from build123d import *

# Parameters (mm, degrees)
SKETCH1_R                     = 3.6195
SKETCH1_R_2                   = 4.7625
SKETCH1_R_3                   = 1.6999966
SKETCH1_W                     = 6.5278
SKETCH1_H                     = 6.5278
BOSS_EXTRUDE1_DEPTH           = 6.35
TAP_DRILL_FOR_6_32_TAP4_D     = 2.7051
TAP_DRILL_FOR_6_32_TAP4_DEPTH = 10.16
TAP_DRILL_FOR_6_32_TAP4_TIP   = 0.81269403
TAP_DRILL_FOR_6_32_TAP3_D     = 2.7051
TAP_DRILL_FOR_6_32_TAP3_DEPTH = 10.16
TAP_DRILL_FOR_6_32_TAP3_TIP   = 0.81269403
SKETCH11_W                    = 6.35
SKETCH11_H                    = 6.1722
BOSS_EXTRUDE2_DEPTH           = 1.016
SKETCH12_W                    = 6.35
SKETCH12_H                    = 6.1722
BOSS_EXTRUDE3_DEPTH           = 1.016
TAP_DRILL_FOR_6_32_TAP1_D     = 2.7051
TAP_DRILL_FOR_6_32_TAP1_DEPTH = 7.62
TAP_DRILL_FOR_6_32_TAP1_TIP   = 0.81269403
TAP_DRILL_FOR_6_32_TAP2_D     = 2.7051
TAP_DRILL_FOR_6_32_TAP2_DEPTH = 7.62
TAP_DRILL_FOR_6_32_TAP2_TIP   = 0.81269403
F_6_CLEARANCE_HOLE1_D         = 3.7973
F_6_CLEARANCE_HOLE1_DEPTH     = 12.7
F_6_CLEARANCE_HOLE1_TIP       = 1.140824014
SKETCH19_R                    = 1.5875
CUT_EXTRUDE1_DEPTH            = 161.894515133
CUT_EXTRUDE2_DEPTH            = 161.894515133


with BuildPart() as part:
    # Sketch1 → Boss-Extrude1 (new body)
    with BuildSketch(Plane(origin=(0, 0, 0), x_dir=(0, 0, -1), z_dir=(1, 0, 0))):
        Polygon((0, 0), (-14.664696837, 25.4), (-144.085303163, 25.4), (-158.75, 0), align=None)
        with Locations((-130.048, 12.7)):
            Circle(SKETCH1_R, mode=Mode.SUBTRACT)
        with Locations((-28.702, 12.7)):
            Circle(SKETCH1_R_2, mode=Mode.SUBTRACT)
        with Locations((-121.5479916, 12.7)):
            Circle(SKETCH1_R_3, mode=Mode.SUBTRACT)
        with Locations((-138.5480084, 12.7)):
            Circle(SKETCH1_R_3, mode=Mode.SUBTRACT)
        with Locations((-79.2861, 12.7889)):
            Rectangle(SKETCH1_W, SKETCH1_H, mode=Mode.SUBTRACT)
    extrude(amount=BOSS_EXTRUDE1_DEPTH)

    # Tap Drill for #6-32 Tap4
    with Locations(Plane(origin=(0, 25.4, 0), x_dir=(1, 0, 0), z_dir=(0, 1, 0))):
        with Locations((3.175, -123.257303163), (3.175, -35.492696837)):
            Hole(TAP_DRILL_FOR_6_32_TAP4_D / 2, depth=TAP_DRILL_FOR_6_32_TAP4_DEPTH)
            with Locations((0, 0, -(TAP_DRILL_FOR_6_32_TAP4_DEPTH + TAP_DRILL_FOR_6_32_TAP4_TIP / 2))):  # 118° drill point
                Cone(0, TAP_DRILL_FOR_6_32_TAP4_D / 2, TAP_DRILL_FOR_6_32_TAP4_TIP, mode=Mode.SUBTRACT)

    # Tap Drill for #6-32 Tap3
    with Locations(Plane(origin=(0, 0, 0), x_dir=(-1, 0, 0), z_dir=(0, -1, 0))):
        with Locations((-3.175, -116.84), (-3.175, -35.56)):
            Hole(TAP_DRILL_FOR_6_32_TAP3_D / 2, depth=TAP_DRILL_FOR_6_32_TAP3_DEPTH)
            with Locations((0, 0, -(TAP_DRILL_FOR_6_32_TAP3_DEPTH + TAP_DRILL_FOR_6_32_TAP3_TIP / 2))):  # 118° drill point
                Cone(0, TAP_DRILL_FOR_6_32_TAP3_D / 2, TAP_DRILL_FOR_6_32_TAP3_TIP, mode=Mode.SUBTRACT)

    # Sketch11 → Boss-Extrude2 (add)
    with BuildSketch(Plane(origin=(0, 68.740766425, 119.0625), x_dir=(1, 0, 0), z_dir=(0, 0.5000000000000038, 0.8660254037844366))):
        with Locations((3.175, -69.9389)):
            Rectangle(SKETCH11_W, SKETCH11_H)
    extrude(amount=BOSS_EXTRUDE2_DEPTH)

    # Sketch12 → Boss-Extrude3 (add)
    with BuildSketch(Plane(origin=(0, 0, 0), x_dir=(-1, 0, 0), z_dir=(0, 0.499999999999998, -0.8660254037844397))):
        with Locations((-3.175, 9.4361)):
            Rectangle(SKETCH12_W, SKETCH12_H)
    extrude(amount=BOSS_EXTRUDE3_DEPTH)

    # Tap Drill for #6-32 Tap1
    with Locations(Plane(origin=(0, 68.740766425, 119.0625), x_dir=(1, 0, 0), z_dir=(0, 0.5000000000000038, 0.8660254037844366))):
        with Locations((3.175, -60.205606325)):
            Hole(TAP_DRILL_FOR_6_32_TAP1_D / 2, depth=TAP_DRILL_FOR_6_32_TAP1_DEPTH)
            with Locations((0, 0, -(TAP_DRILL_FOR_6_32_TAP1_DEPTH + TAP_DRILL_FOR_6_32_TAP1_TIP / 2))):  # 118° drill point
                Cone(0, TAP_DRILL_FOR_6_32_TAP1_D / 2, TAP_DRILL_FOR_6_32_TAP1_TIP, mode=Mode.SUBTRACT)

    # Tap Drill for #6-32 Tap2
    with Locations(Plane(origin=(0, 0, 0), x_dir=(-1, 0, 0), z_dir=(0, 0.49999999999999806, -0.8660254037844398))):
        with Locations((-3.175, 19.169393675)):
            Hole(TAP_DRILL_FOR_6_32_TAP2_D / 2, depth=TAP_DRILL_FOR_6_32_TAP2_DEPTH)
            with Locations((0, 0, -(TAP_DRILL_FOR_6_32_TAP2_DEPTH + TAP_DRILL_FOR_6_32_TAP2_TIP / 2))):  # 118° drill point
                Cone(0, TAP_DRILL_FOR_6_32_TAP2_D / 2, TAP_DRILL_FOR_6_32_TAP2_TIP, mode=Mode.SUBTRACT)

    # #6 Clearance Hole1
    with Locations(Plane(origin=(0, 25.4, 0), x_dir=(1, 0, 0), z_dir=(0, 1, 0))):
        with Locations((3.175, -79.375)):
            Hole(F_6_CLEARANCE_HOLE1_D / 2, depth=F_6_CLEARANCE_HOLE1_DEPTH)
            with Locations((0, 0, -(F_6_CLEARANCE_HOLE1_DEPTH + F_6_CLEARANCE_HOLE1_TIP / 2))):  # 118° drill point
                Cone(0, F_6_CLEARANCE_HOLE1_D / 2, F_6_CLEARANCE_HOLE1_TIP, mode=Mode.SUBTRACT)

    # Sketch19 → Cut-Extrude1 (cut, through all)
    with BuildSketch(Plane.ZY):
        with Locations((151.13, 3.81)):
            Circle(SKETCH19_R)
        with Locations((7.62, 3.81)):
            Circle(SKETCH19_R)
    extrude(amount=-CUT_EXTRUDE1_DEPTH, mode=Mode.SUBTRACT)

    # Sketch20 → Cut-Extrude2 (cut, through all)
    with BuildSketch(Plane.ZY):
        Polygon((64.373574984, 7.366), (39.116, 17.286492924), (39.116, 7.366), align=None)
        Polygon((69.4182, 18.034), (44.160625016, 18.034), (69.4182, 8.113507076), align=None)
        Polygon((112.039277302, 7.366), (89.195364135, 17.488514329), (89.195364135, 7.366), align=None)
        Polygon((115.824, 18.034), (92.980086833, 18.034), (115.824, 7.911485671), align=None)
    extrude(amount=-CUT_EXTRUDE2_DEPTH, mode=Mode.SUBTRACT)


solid = part.part
Can you work these out from the model? Positions are in its coordinate system, mm. A direction names the side the tool comes from. Coordinates: 2 decimals unless noted, no trailing zeros. Loops run counter-clockwise (first coordinate to the right, second up) from the corner with the lowest first, then second, coordinate; pieces in that order, holes last. Notation, with made-up numbers: (22.25, 35.25) - (39.25, 35.25) arc R27 cw to (39.25, 73.25) - close; hole circle Ø7 at (88.25, 28.5). An arc over 180 degrees is marked (long way). Answer as a JSON object with one key per item and string values. Group by question number.
Item 1: If we section it at C-C (z = 7.62): List the corners of the cut face in (x, y) for me.
Item 2: For pin 1 (3 mm diameter, centred on x = 4.5, y = 15, fed in from +Z); pin 2 (1.9 mm diameter, centred on x = 3.5, y = 12, fed in from +Z); pin 3 (2.5 mm diameter, centred on x = 3.18, z = 35.49, fed in from +Y), each with a flat end and sliding along its axis, tell me the tip position at first contact or that it passes through.
Item 3: On a 3-axis mill with a long thin cutter (end or side, diameter ignored), from which of +Z, -Z, +X, -X, +Y, -Y can I reach the whole of each face in a straight line? I mean faces 1 (the face through (2.88, 5.15, 118.16)), 2 (the face through (3.587, 20.661, 81.229)), 3 (the face through (3, 0, 80)), 4 (the face through (5, 16.053, 81)). Say none if no direction works.
Item 4: If we section it at D-D (z = 102.5): List the corners of the cut face in (x, y) for me, plus the area to 3 significant figures.
Item 5: If we section it at A-A (z = 52.5): List the corners of the cut face in (x, y) for me, plus the area to 3 significant figures.
Item 6: If we section it at B-B (y = 21.75): List the corners of the cut face in (x, z) for me (3 decimals).
Item 7: If I drill on L1, parallel to Z at x = 5.25, y = 4; L2, parallel to Y at x = 3, z = 58; L3, parallel to Z at x = 1.5, y = 2.5, over which ranges is the centre line in solid material (lowest first)? Write a range as from..to.
Item 8: If we mould it in two halves opening along Z, with no side actions, what happens to faces 5 (the face through (3.13, 2.79, 157.14)), 6 (the face through (0, 7, 80)), 7 (the face through (3, 18.034, 57))? For each: released by +Z, released by -Z, zero draft, split by the parting line, or undercut.
Returned:
{
 "1": {"outline": "(0, 0) - (6.35, 0) - (6.35, 2.22) - (0, 2.22) - close; (0, 5.4) - (6.35, 5.4) - (6.35, 13.2) - (0, 13.2) - close"},
 "2": {"pin 1": "stops at z = 150.96", "pin 2": "stops at z = 153.54", "pin 3": "stops at y = 15.18"},
 "3": {"face 1": "-Y", "face 2": "+Y", "face 3": "+Z, -Z, +X, -X, -Y", "face 4": "+X, -X"},
 "4": {"outline": "(0, 0) - (6.35, 0) - (6.35, 7.37) - (0, 7.37) - close; (0, 11.59) - (6.35, 11.59) - (6.35, 13.82) - (0, 13.82) - close; (0, 18.03) - (6.35, 18.03) - (6.35, 25.4) - (0, 25.4) - close", "area": "108 mm²"},
 "5": {"outline": "(0, 0) - (6.35, 0) - (6.35, 7.37) - (0, 7.37) - close; (0, 12.03) - (6.35, 12.03) - (6.35, 14.76) - (0, 14.76) - close; (0, 18.03) - (6.35, 18.03) - (6.35, 25.4) - (0, 25.4) - close", "area": "111 mm²"},
 "6": {"outline": "(0, 12.557) - (6.35, 12.557) - (6.35, 146.193) - (0, 146.193) - close; hole circle Ø3.797 at (3.175, 79.375); hole circle Ø2.705 at (3.175, 35.493); hole circle Ø2.705 at (3.175, 123.257)"},
 "7": {"L1": "z = 2.31..6.04, 9.2..149.55, 152.71..156.44", "L2": "y = 0..7.37, 9.87..12.6, 18.03..25.4", "L3": "z = 1.44..6.72, 8.52..150.23, 152.03..157.31"},
 "8": {"face 5": "released by +Z", "face 6": "zero draft", "face 7": "undercut"}
}
